Input: part model. Units: mm. Frame: model coordinates. A direction names the side the tool comes from. Give positions to 0.01 mm unless a question says otherwise; leave off trailing zeros. Loops run counter-clockwise (first coordinate to the right, second up) from the corner with the lowest first, then second, coordinate; pieces in that order, holes last. Notation, with made-up numbers: M -4,34 L 42,34 A27 ccw 42,60 Z; hole C 5,-24 d1. An arc over 180 degrees is marked long. One line per item, written item: value. Start each with the question number.
(1) Pull-direction query (X, two-part tool) for faces 3 (the flat face through (-3, 2, 5.5)), 4 (the cylindrical face through (-2.539, -1.947, 2.712)), 5 (the flat face through (10, 0, 11)), 6 (the flat face through (-3, 6, 25)); classes: released by +X, released by -X, zero draft, split by the parting line, or undercut.
(2) Pin query (flat end, axial travel): P1, Ø4.5, axis at x = -0.5, y = 1, coming from the +Z side; P2, Ø5, axis at x = -0.5, y = 3, coming from the +Z side. Return the tip coordinate at first contact, or that it passes through.
(3) Ray query, line 1 along X through (y, z) = (0, 2.7); line 2 along Y through (x, z) = (0, 15.25). Return the intervals inside material, ascending. Write a range as from..to.
(4) Section D-D on z = 3.5. Output: boundary loops of the cut face in (x, y).
(5) Section B-B on z = 13. Output: boundary loops of the cut face in (x, y).
(6) Section A-A on y = 0. Output: boundary loops of the cut face in (x, z), plus the area to 3 significant figures.
(7) Access query for faces 1 (the flat face through (-10, 0, 11)), 2 (the cylindrical face through (-1.16, -5.223, 15.372)). Directions: +Z, -Z, +X, -X, +Y, -Y. A direction counts if a zero-diameter tool reaches every point of the face in a straight line with its end or side. Return the directions, or none.
```python
from build123d import *

# Parameters (mm, degrees)
SKETCH1_R           = 3.2
BOSS_EXTRUDE1_DEPTH = 25
FILLET1_R           = 3
SKETCH2_R           = 5.35
CUT_EXTRUDE1_DEPTH  = 19.5
FILLET2_R           = 1
FILLET3_R           = 1


with BuildPart() as part:
    # Sketch1 → Boss-Extrude1 (new body)
    with BuildSketch(Plane.XY):
        with BuildLine():
            Line((-7, -10), (7, -10))
            ThreePointArc((7, -10), (9.121320344, -9.121320344), (10, -7))
            Line((10, -7), (10, 7))
            ThreePointArc((10, 7), (9.121320344, 9.121320344), (7, 10))
            Line((7, 10), (-7, 10))
            ThreePointArc((-7, 10), (-9.121320344, 9.121320344), (-10, 7))
            Line((-10, 7), (-10, -7))
            ThreePointArc((-10, -7), (-9.121320344, -9.121320344), (-7, -10))
        make_face()
        Circle(SKETCH1_R, mode=Mode.SUBTRACT)
    extrude(amount=BOSS_EXTRUDE1_DEPTH)

    # Fillet1
    fillet1_edges = [part.edges().sort_by_distance(p)[0] for p in [
        (9.121320344, 9.121320344, 25),
        (0, 10, 25),
        (-9.121320344, 9.121320344, 25),
        (-10, 0, 25),
        (-9.121320344, -9.121320344, 25),
        (0, -10, 25),
        (9.121320344, -9.121320344, 25),
        (10, 0, 25),
    ]]
    fillet(fillet1_edges, radius=FILLET1_R)

    # Sketch2 → Cut-Extrude1 (cut)
    with BuildSketch(Plane.XY.offset(25)):
        Circle(SKETCH2_R)
    extrude(amount=-CUT_EXTRUDE1_DEPTH, mode=Mode.SUBTRACT)

    # Fillet2
    fillet2_edges = [part.edges().sort_by_distance(p)[0] for p in [
        (-5.35, 0, 25),
    ]]
    fillet(fillet2_edges, radius=FILLET2_R)

    # Fillet3
    fillet3_edges = [part.edges().sort_by_distance(p)[0] for p in [
        (-5.35, 0, 5.5),
    ]]
    fillet(fillet3_edges, radius=FILLET3_R)


solid = part.part
```
Output values:
1. face 3: undercut
1. face 4: undercut
1. face 5: released by +X
1. face 6: zero draft
2. P1: stops at z = 5.5
2. P2: stops at z = 24.59
3. line 1: x = -10..-3.2, 3.2..10
3. line 2: y = -10..-5.35, 5.35..10
4. outline: M -10,-7 A3 ccw -7,-10 L 7,-10 A3 ccw 10,-7 L 10,7 A3 ccw 7,10 L -7,10 A3 ccw -10,7 Z; hole C 0,0 d6.4
5. outline: M -10,-7 A3 ccw -7,-10 L 7,-10 A3 ccw 10,-7 L 10,7 A3 ccw 7,10 L -7,10 A3 ccw -10,7 Z; hole C 0,0 d10.7
6. outline: M -10,0 L -3.2,0 L -3.2,5.5 L -4.35,5.5 A1 cw -5.35,6.5 L -5.35,24 A1 ccw -6.35,25 L -7,25 A3 ccw -10,22 Z; M 3.2,0 L 10,0 L 10,22 A3 ccw 7,25 L 6.35,25 A1 ccw 5.35,24 L 5.35,6.5 A1 cw 4.35,5.5 L 3.2,5.5 Z
6. area: 252 mm²
7. face 1: +Z, -Z, -X, +Y, -Y
7. face 2: +Z
